Build history of the part. All positions in model axes, mm. A direction names the side the tool comes from. Round coordinates to 2 decimals unless told otherwise and drop trailing zeros. Write each loop counter-clockwise with the first axis right and the second up, starting at its lowest first coordinate (ties: lowest second). Pieces come first, ordered by that corner, then holes.
1) Wall check: probe 1 along Z at (x, y) = (-11, -9.25); probe 2 along Z at (x, y) = (-5, -1.15); probe 3 along Y at (x, z) = (-3.75, 3.5). Give the ranges that are in metal, low to high.
2) Saw through at D-D (y = -11.25). Write the cut outline in (x, z).
3) Saw through at C-C (x = -9). Write the cut outline in (y, z), plus the area to 3 significant figures.
4) Pull direction Y, two halves, no side cores. Call faces 5 (the cylindrical face through (-4.492, -1.479, -9.636)), 6 (the flat face through (-7, -5, 3)), 7 (the flat face through (-4.1, -13, 1.4)): +Y half, -Y half, draft (parallel to the pull), parting line (faces both ways), or undercut.
5) Which spindle directions (+Z, -Z, +X, -X, +Y, -Y) get a long thin tool onto all of the face, cutting with end or side? Do faces 1 (the flat face through (0, -6, 1.323)), 2 (the flat face through (-8, -8, -1)), 3 (the flat face through (-8, -8, 5)), 4 (the flat face through (-8, -8, -5)). Say none if no direction does.
6) Saw through at B-B (z = 0). Write the cut outline in (x, y), plus the area to 3 significant figures.
7) Saw through at A-A (y = -9). Write the cut outline in (x, z).
8) Flat gauge pins, fed straight in: pin 1 (6 mm diameter, centred on x = -3.5, y = -7, fed in from +Z); pin 2 (3 mm diameter, centred on x = -7, y = -8.5, fed in from +Z); pin 3 (5 mm diameter, centred on x = 0.5, z = 8, fed in from +Y); pin 4 (0.6 mm diameter, centred on y = -3.5, z = 4, fed in from -X). Where does each tip first touch, or does it go through?
from build123d import *

# Parameters (mm, degrees)
F0_R      = 14
F0_R_2    = 1.1
F1_DEPTH  = 3
F3_DEPTH  = 10
F5_DEPTH  = 13.001
F6_W      = 14
F6_H      = 2
F7_DEPTH  = 6
F8_W      = 14
F8_H      = 2
F9_DEPTH  = 8
F10_R     = 3
F11_DEPTH = 10
F12_R     = 5
F13_R     = 5
F14_R     = 1.1
F15_DEPTH = 19.001


# Not quite as in the source:
# - a feature names something its author has since deleted; it is built from what else it names


with BuildPart() as f1:
    # F0 (on Front) → F1 (new body)
    with BuildSketch(Plane.XZ):
        Circle(F0_R)
        with Locations((-5, -8.6602540378)):
            Circle(F0_R_2, mode=Mode.SUBTRACT)
        with Locations((-5, 8.6602540378)):
            Circle(F0_R_2, mode=Mode.SUBTRACT)
        with Locations((10, 0)):
            Circle(F0_R_2, mode=Mode.SUBTRACT)
    extrude(amount=F1_DEPTH)

    # F2 (on face) → F3 (join)
    with BuildSketch(Plane.XZ.offset(3)):
        with BuildLine():
            ThreePointArc((-3.3166247904, -5), (-1.7320508076, -5.7445626465), (0, -6))
            ThreePointArc((0, -6), (6, 0), (0, 6))
            ThreePointArc((0, 6), (-1.7320508076, 5.7445626465), (-3.3166247904, 5))
            Line((-3.3166247904, 5), (-13.0766968306, 5))
            ThreePointArc((-13.0766968306, 5), (-14, 0), (-13.0766968306, -5))
            Line((-13.0766968306, -5), (-3.3166247904, -5))
        make_face()
    extrude(amount=F3_DEPTH)

    # F4 (on face) → F5 (cut, through all)
    with BuildSketch(Plane(origin=(0, 0, 0), x_dir=(-1, 0, 0), z_dir=(0, 1, 0))):
        with BuildLine():
            Line((1.5, 1.3228756555), (-1.5, 1.3228756555))
            ThreePointArc((-1.5, 1.3228756555), (0, -2), (1.5, 1.3228756555))
        make_face()
    extrude(amount=-F5_DEPTH, mode=Mode.SUBTRACT)

    # F6 (on face) → F7 (cut, symmetric)
    with BuildSketch(Plane.XY.offset(5)):
        with Locations((-7, -4)):
            Rectangle(F6_W, F6_H)
    extrude(amount=F7_DEPTH, both=True, mode=Mode.SUBTRACT)

    # F8 (on face) → F9 (cut)
    with BuildSketch(Plane.XZ.offset(13)):
        with Locations((-7, 0)):
            Rectangle(F8_W, F8_H)
    extrude(amount=-F9_DEPTH, mode=Mode.SUBTRACT)

    # F10 (on face) → F11 (cut)
    with BuildSketch(Plane.XZ.offset(3)):
        with Locations((-5, 8.6602540378)):
            Circle(F10_R)
    extrude(amount=F11_DEPTH, mode=Mode.SUBTRACT)

    # F12
    f12_edges = [f1.edges().sort_by_distance(p)[0] for p in [
        (-3.316625, -9, 5),
    ]]
    fillet(f12_edges, radius=F12_R)

    # F13
    f13_edges = [f1.edges().sort_by_distance(p)[0] for p in [
        (-3.316625, -8, -5),
    ]]
    fillet(f13_edges, radius=F13_R)

    # F14 (on face) → F15 (cut, through all)
    with BuildSketch(Plane.XY.offset(5)):
        with Locations((-9, -9)):
            Circle(F14_R)
    extrude(amount=-F15_DEPTH, mode=Mode.SUBTRACT)


solid = f1.part
Evaluation:
1. probe 1: z = -5 to -1, 1 to 5
1. probe 2: z = -13.08 to -9.76, -7.56 to 7.56, 9.76 to 13.08
1. probe 3: y = -13 to -5, -3 to 0
2. outline: (-13.96, -1) arc R14 ccw to (-13.08, -5) - (-4.58, -5) arc R5 cw to (-2.5, -5.45) arc R6 ccw (long way) to (-2.5, 5.45) arc R5 cw to (-4.58, 5) - (-13.08, 5) arc R14 ccw to (-13.96, 1) - (-1.73, 1) arc R2 cw to (-1.5, 1.32) - (1.5, 1.32) arc R2 cw (long way) to (-1.73, -1) - close
3. outline: (-13, -5) - (-10.1, -5) - (-10.1, -1) - (-13, -1) - close; (-13, 1) - (-10.1, 1) - (-10.1, 5) - (-13, 5) - close; (-7.9, -5) - (-3, -5) - (-3, -10.72) - (0, -10.72) - (0, 10.72) - (-3, 10.72) - (-3, -1) - (-7.9, -1) - close; (-7.9, 1) - (-5, 1) - (-5, 5) - (-7.9, 5) - close
3. area: 119 mm2
4. face 5: draft
4. face 6: undercut
4. face 7: -Y half
5. face 1: +Y, -Y
5. face 2: -X, -Y
5. face 3: +Z, -X, -Y
5. face 4: -Z, -X, -Y
6. outline: (-14, -3) - (-2, -3) - (-2, 0) - (-14, 0) - close; (2, -13) - (6, -13) - (6, -3) - (8.9, -3) - (8.9, 0) - (2, 0) - close; (11.1, -3) - (14, -3) - (14, 0) - (11.1, 0) - close
6. area: 105 mm2
7. outline: (-13.96, -1) arc R14 ccw to (-13.08, -5) - (-10.1, -5) - (-10.1, -1) - close; (-13.96, 1) - (-10.1, 1) - (-10.1, 5) - (-13.08, 5) arc R14 ccw to start; (-7.9, -5) - (-4.58, -5) arc R5 cw to (-2.5, -5.45) arc R6 ccw (long way) to (-2.5, 5.45) arc R5 cw to (-4.58, 5) - (-7.9, 5) - (-7.9, 1) - (-1.73, 1) arc R2 cw to (-1.5, 1.32) - (1.5, 1.32) arc R2 cw (long way) to (-1.73, -1) - (-7.9, -1) - close
8. pin 1: stops at z = 5.98
8. pin 2: stops at z = 5
8. pin 3: stops at y = 0
8. pin 4: stops at x = 0
